Job drawing, mm, ordinate dimensions from the low corner. One solid piece. A direction names the side the tool comes from. Give positions to 0.01 mm unless a question says otherwise; leave off trailing zeros. Loops run counter-clockwise (first coordinate to the right, second up) from the corner with the lowest first, then second, coordinate; pieces in that order, holes last. Notation, with made-up numbers: M 83,-20 L 91,-20 A27 ccw 91,-4 Z; hole C 12,-40 d7. An arc over 180 degrees is marked long. Put each result on its own line as item: value.
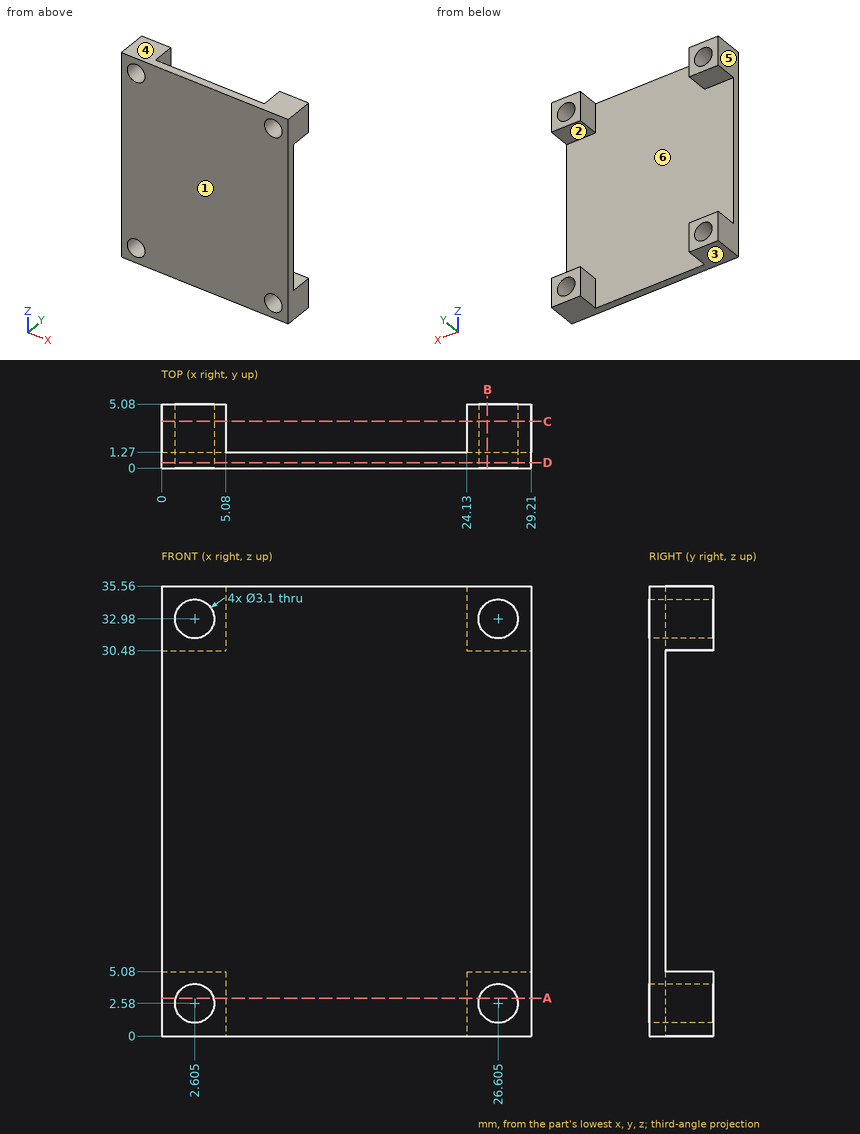
Q1. Slice it at B-B (x = 25.75). List the corners of the cut face in (y, z), and give its area (3 significant figures).
Here are the results:
outline: M 0,0 L 5.08,0 L 5.08,1.29 L 0,1.29 Z; M 0,3.87 L 5.08,3.87 L 5.08,5.08 L 1.27,5.08 L 1.27,30.48 L 5.08,30.48 L 5.08,31.69 L 0,31.69 Z; M 0,34.27 L 5.08,34.27 L 5.08,35.56 L 0,35.56 Z
area: 57.6 mm²
Q2. Probe line 1 (Z direction, x = 26.75, y = 3.75); line 2 (X direction, y = 2.6, z = 34); line 3 (Z direction, x = 25, y = 2.65). List the from-to ranges inside material, lowest first. Write a range as from..to.
Here are the results:
line 1: 0..1.04, 4.12..5.08, 30.48..31.44, 34.52..35.56
line 2: 0..1.44, 3.77..5.08, 24.13..25.44, 27.77..29.21
line 3: 0..5.08, 30.48..35.56
Q3. Slice it at A-A (z = 3). List the corners of the cut face in (x, y), and give its area (3 significant figures).
Here are the results:
outline: M 0,0 L 1.11,0 L 1.11,5.08 L 0,5.08 Z; M 4.1,0 L 25.11,0 L 25.11,5.08 L 24.13,5.08 L 24.13,1.27 L 5.08,1.27 L 5.08,5.08 L 4.1,5.08 Z; M 28.1,0 L 29.21,0 L 29.21,5.08 L 28.1,5.08 Z
area: 45.5 mm²
Q4. Drop flat-ended pins along their axis: pin 1 Ø1.9 at (x, z) = (2.6, 32.98) entering from +Y; pin 2 Ø1.5 at (x, z) = (26, 22) entering from +Y. Give the stop position or say it passes through.
Here are the results:
pin 1: through
pin 2: y = 1.27
Q5. Slice it at D-D (y = 0.45). List the corners of the cut face in (x, z) (3 decimals).
Here are the results:
outline: M 0,0 L 29.21,0 L 29.21,35.56 L 0,35.56 Z; hole C 2.605,2.58 d3.1; hole C 2.605,32.98 d3.1; hole C 26.605,2.58 d3.1; hole C 26.605,32.98 d3.1
Q6. Slice it at C-C (y = 3.7). List the corners of the cut face in (x, z) (3 decimals), and give its area (3 significant figures).
Here are the results:
outline: M 0,0 L 5.08,0 L 5.08,5.08 L 0,5.08 Z; M 0,30.48 L 5.08,30.48 L 5.08,35.56 L 0,35.56 Z; M 24.13,0 L 29.21,0 L 29.21,5.08 L 24.13,5.08 Z; M 24.13,30.48 L 29.21,30.48 L 29.21,35.56 L 24.13,35.56 Z; hole C 2.605,2.58 d3.1; hole C 2.605,32.98 d3.1; hole C 26.605,2.58 d3.1; hole C 26.605,32.98 d3.1
area: 73.0 mm²
Q7. Mould opens along Z. For the marked faces 3, 4, 5 and 6 say: pulls with the +Z half, pulls with the -Z half, needs draft (parallel to the pull), parting line crosses it, or undercut.
Here are the results:
face 3: pulls with the -Z half
face 4: pulls with the +Z half
face 5: needs draft
face 6: undercut
Q8. Tool access for the marked faces 1 and 2: list every direction of +Z, -Z, +X, -X, +Y, -Y with a clear straight run to the whole face (end or side of a thin tool).
Here are the results:
face 1: +Z, -Z, +X, -X, -Y
face 2: +X, -X, +Y
